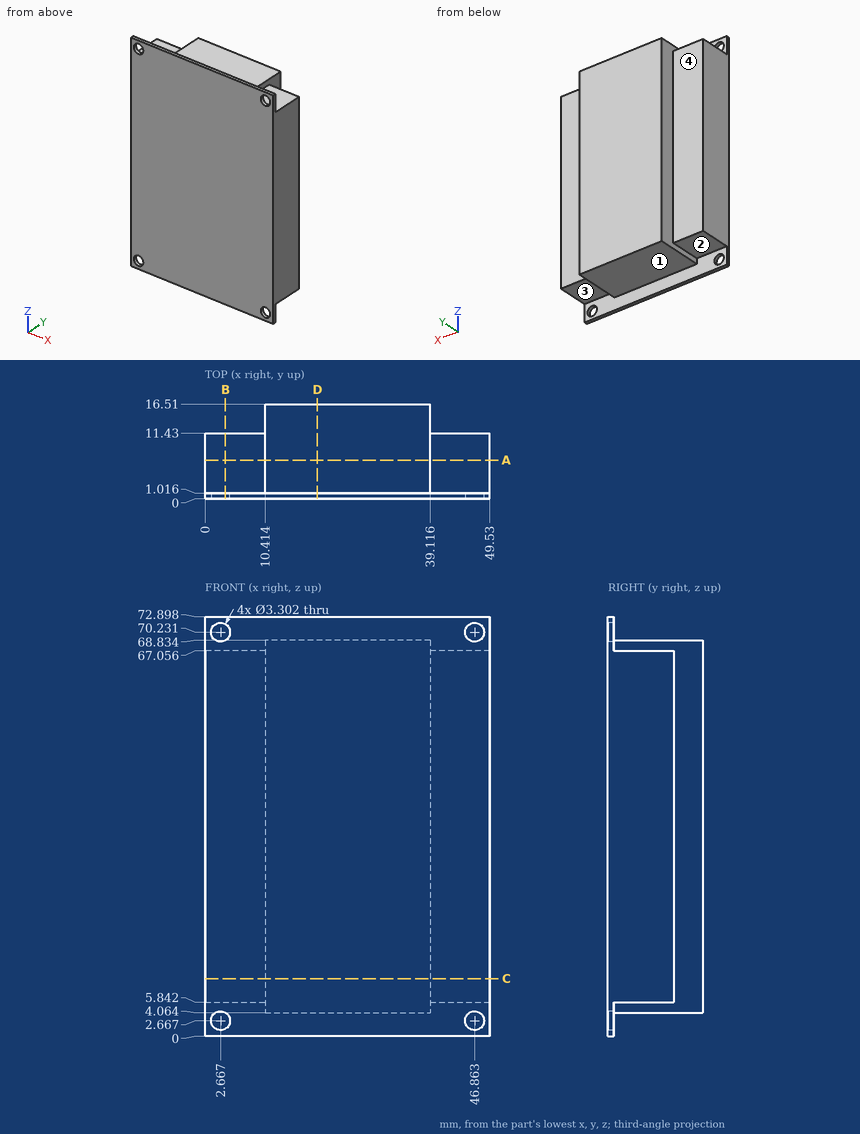
Can you work these out from the drawing? Everything is in mm from the part's minimum corner. A direction names the side the tool comes from. Round coordinates to 2 decimals unless told otherwise and drop trailing zeros. Loops run counter-clockwise (first coordinate to the right, second up) from the corner with the lowest first, then second, coordinate; pieces in that order, holes last. Notation, with made-up numbers: M -33,60 L -13,60 A13 cw -13,67 Z; hole C 33,3.5 d2. An arc over 180 degrees is marked long. Write item = value, one per line.
1. I want a section at A-A, the plane y = 6.75. Write out the boundary of the cut face in (x, z), and give its area (3 significant figures).
Results below:
outline = M 0,5.84 L 10.41,5.84 L 10.41,4.06 L 39.12,4.06 L 39.12,5.84 L 49.53,5.84 L 49.53,67.06 L 39.12,67.06 L 39.12,68.83 L 10.41,68.83 L 10.41,67.06 L 0,67.06 Z
area = 3,130 mm²
2. I want a section at C-C, the plane z = 10. Write out the boundary of the cut face in (x, y).
Results below:
outline = M 0,0 L 49.53,0 L 49.53,11.43 L 39.12,11.43 L 39.12,16.51 L 10.41,16.51 L 10.41,11.43 L 0,11.43 Z
3. Will these pins go through, and if not, where does the flat tip stop? P1, Ø12, axis at x = 37, z = 14, coming from the -Y side; P2, Ø3, axis at x = 6, z = 26, coming from the +Y side; P3, Ø2, axis at x = 46.863, z = 2.667, coming from the -Y side; P4, Ø5, axis at x = 27, y = 11, coming from the -Z side.
Results below:
P1 = 0
P2 = 11.43
P3 = through
P4 = 4.06
4. Which directions (+Z, -Z, +X, -X, +Y, -Y) give clear straight access to the entire face, cutting with the end or side of a thin tool? Please do the marked faces 1, 2, 3 and 4.
Results below:
face_1 = -Z, +X, -X, +Y
face_2 = -Z, -X, +Y
face_3 = -Z, +X, +Y
face_4 = +Z, -Z, -X, +Y
5. I need wall thicknesses on probe 1 along Z at (x, y) = (32, 5.5); probe 2 along Z at (x, y) = (7.5, 2.75); probe 3 along X at (y, z) = (14.5, 12.5). Which ranges of each line are inside material? Lowest first, please.
Results below:
probe_1 = 4.06 to 68.83
probe_2 = 5.84 to 67.06
probe_3 = 10.41 to 39.12
6. I want a section at B-B, the plane x = 3.5. Write out the boundary of the cut face in (y, z), and give its area (3 significant figures).
Results below:
outline = M 0,0 L 1.02,0 L 1.02,1.24 L 0,1.24 Z; M 0,4.09 L 1.02,4.09 L 1.02,5.84 L 11.43,5.84 L 11.43,67.06 L 1.02,67.06 L 1.02,68.81 L 0,68.81 Z; M 0,71.66 L 1.02,71.66 L 1.02,72.9 L 0,72.9 Z
area = 706 mm²
7. I want a section at D-D, the plane x = 19.5. Write out the boundary of the cut face in (y, z).
Results below:
outline = M 0,0 L 1.02,0 L 1.02,4.06 L 16.51,4.06 L 16.51,68.83 L 1.02,68.83 L 1.02,72.9 L 0,72.9 Z
